```python
from build123d import *

# Parameters (mm, degrees)
SKETCH_1_R           = 7
SKETCH_1_R_2         = 2.5
EXTRUDE_1_DEPTH      = 22
MM_1_REACH           = 25.055
MM_1_BORE_R          = 2
MM_1_ON_FACE_2_REACH = 25.854
MM_1_BORE_2_R        = 2


with BuildPart() as part:
    # 草图1 → 凸台-拉伸1 (new body)
    with BuildSketch(Plane(origin=(0, 0, 0), x_dir=(1, 0, 0), z_dir=(0, 1, 0))):
        with Locations(Location((0, 0, 0), (0, 0, 270))):
            Circle(SKETCH_1_R)
        with Locations(Location((0, 0, 0), (0, 0, 270))):
            Circle(SKETCH_1_R_2, mode=Mode.SUBTRACT)
    extrude(amount=EXTRUDE_1_DEPTH)

    # 大小mm 暗销孔1 bore (on position points) → 大小mm 暗销孔1 (cut, up to next)
    with BuildSketch(Plane(origin=(3.857759844, 15.771125488, 5.841034924), x_dir=(0.834433560595, 0, -0.551108549156), z_dir=(0.551108549156, 0, 0.834433560595)), mode=Mode.PRIVATE) as mm_1_sk1:
        Circle(MM_1_BORE_R)
    mm_1_tool1 = extrude(mm_1_sk1.sketch, amount=-MM_1_REACH, mode=Mode.PRIVATE) & part.part
    add(mm_1_tool1.solids().sort_by_distance((3.85776, 15.771125, 5.841035))[0], mode=Mode.SUBTRACT)

    # 大小mm 暗销孔1 bore 2 (on position points) → 大小mm 暗销孔1 on face 2 (cut, up to next)
    with BuildSketch(Plane(origin=(3.760299327, 5.067053502, 5.904248383), x_dir=(0.843463865935, 0, -0.537185914616), z_dir=(0.537185914616, 0, 0.843463865935)), mode=Mode.PRIVATE) as mm_1_on_face_2_sk1:
        Circle(MM_1_BORE_2_R)
    mm_1_on_face_2_tool1 = extrude(mm_1_on_face_2_sk1.sketch, amount=-MM_1_ON_FACE_2_REACH, mode=Mode.PRIVATE) & part.part
    add(mm_1_on_face_2_tool1.solids().sort_by_distance((3.760299, 5.067054, 5.904248))[0], mode=Mode.SUBTRACT)


solid = part.part
```
Design review of the part built by this model. Coordinates are the model's own, in mm. Give positions to 0.01 mm unless a question says otherwise; leave off trailing zeros. Order: outer loops, then holes, each group sorted by start corner. A loop starts at its lowest first (then second) coordinate and runs counter-clockwise, first axis right, second up. Notation, with made-up numbers: M 22,28 L 51,28 A24 cw 51,42 Z; hole C 81,-11 d2. An arc over 180 degrees is marked long. One line per question, with ' | ' between items. Start each with the question number.
Q1. The part is to be moulded in two halves that separate along Z. For faces 1 (the face through (3.96, 16.37, 2.53)), 2 (the face through (0, 22, 3)), 3 (the face through (-4.259, 10.846, -5.555)), say which applies: +Z half, -Z half, draft (parallel to the pull), parting line (faces both ways), or undercut.
Q2. We need section C-C (y = 11.75). Write out the cut boundary in (x, z), plus the area to 3 significant figures.
Q3. We need section D-D (x = 5.75). Write out the cut boundary in (y, z), plus the area to 3 significant figures.
Q4. We need section B-B (z = -1.25). Write out the cut boundary in (x, y), plus the area to 3 significant figures.
Q5. For L1, parallel to Y at x = 4.25, z = 3.5; L2, parallel to X at y = 17.75, z = 0; L3, parallel to Y at x = 4.25, z = 3.75, list the stretches that pass through material, from the lowest coordinate up. Write a range as [from, to].
Q6. For pin 1 Ø5 at (y, z) = (8.5, 0.5) entering from +X; pin 2 Ø1 at (x, y) = (-3, 6) entering from +Z; pin 3 Ø4.5 at (x, z) = (0, 0) entering from +Y; pin 4 Ø4 at (x, y) = (-4, 10) entering from -Z, all flat-tipped, find the tip position at first contact; note any pin that passes through.
Q7. We need section A-A (x = -1.75). Write out the cut boundary in (y, z), plus the area to 3 significant figures.
Returned:
1) face 1: undercut | face 2: draft | face 3: parting line
2) outline: C 0,0 d14; hole C 0,0 d5 | area: 134 mm2
3) outline: M 0,-3.99 L 22,-3.99 L 22,3.99 L 0,3.99 Z | area: 176 mm2
4) outline: M -6.89,0 L -2.17,0 L -2.17,22 L -6.89,22 Z; M 2.17,0 L 6.89,0 L 6.89,22 L 2.17,22 Z | area: 208 mm2
5) L1: [0, 4.02], [6.11, 14.59], [16.95, 22] | L2: [-7, -2.5], [2.5, 7] | L3: [0, 3.83], [6.31, 14.43], [17.12, 22]
6) pin 1: x = 7 | pin 2: z = 6.54 | pin 3: through | pin 4: z = -6.71
7) outline: M 0,-6.78 L 22,-6.78 L 22,-1.79 L 0,-1.79 Z; M 0,1.79 L 22,1.79 L 22,6.78 L 0,6.78 Z | area: 220 mm2
